```python
from build123d import *

# Parameters (mm, degrees)
ESQUISSE1_W        = 20
ESQUISSE1_H        = 5
BOSS_EXTRU_1_DEPTH = 5


with BuildPart() as part:
    # Esquisse1 → Boss.-Extru.1 (new body)
    with BuildSketch(Plane.XY):
        Polygon((-100, 150), (100, 150), (100, 75), (105, 75), (105, 150), (113, 150), (113, 0), (-113, 0), (-113, 150), (-105, 150), (-105, 75), (-100, 75), align=None)
        with Locations((83, 7.5)):
            Rectangle(ESQUISSE1_W, ESQUISSE1_H, mode=Mode.SUBTRACT)
        with Locations((83, 57.5)):
            Rectangle(ESQUISSE1_W, ESQUISSE1_H, mode=Mode.SUBTRACT)
        Polygon((-15, 5), (15, 5), (15, 10), (0, 10), (-15, 10), align=None, mode=Mode.SUBTRACT)
        Polygon((-15, 60), (0, 60), (15, 60), (15, 55), (-15, 55), align=None, mode=Mode.SUBTRACT)
        with Locations((-83, 7.5)):
            Rectangle(ESQUISSE1_W, ESQUISSE1_H, mode=Mode.SUBTRACT)
        with Locations((-83, 57.5)):
            Rectangle(ESQUISSE1_W, ESQUISSE1_H, mode=Mode.SUBTRACT)
    extrude(amount=BOSS_EXTRU_1_DEPTH)


solid = part.part
```
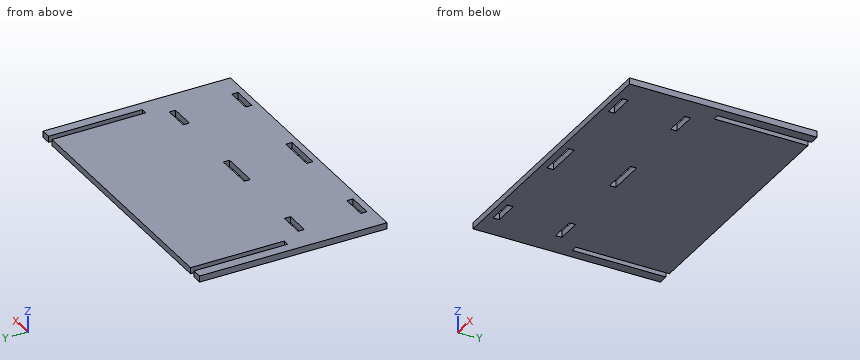
The model under review builds one solid part; all positions refer to its coordinate system, in mm. Round coordinates to 2 decimals unless told otherwise and drop trailing zeros. Loops run counter-clockwise (first coordinate to the right, second up) from the corner with the lowest first, then second, coordinate; pieces in that order, holes last. Notation, with made-up numbers: M 55.5,56.5 L 60.5,56.5 A30 ccw 60.5,90.5 Z; hole C 68.25,-16.75 d3. An arc over 180 degrees is marked long. Answer as a JSON object with one key per item and string values.
(1) Take a section at B-B on x = 83.5. Give the boundary of the cut face in (y, z), and give its area (3 significant figures).
Resolved:
{"outline": "M 0,0 L 5,0 L 5,5 L 0,5 Z; M 10,0 L 55,0 L 55,5 L 10,5 Z; M 60,0 L 150,0 L 150,5 L 60,5 Z", "area": "700 mm²"}
(2) Take a section at A-A on y = 114. Give the boundary of the cut face in (x, z).
Resolved:
{"outline": "M -113,0 L -105,0 L -105,5 L -113,5 Z; M -100,0 L 100,0 L 100,5 L -100,5 Z; M 105,0 L 113,0 L 113,5 L 105,5 Z"}
(3) To check wall thickness, follow line 1 along X through (y, z) = (59, 1.5); line 2 along Y through (x, z) = (9, 1.2); line 3 along X through (y, z) = (115, 0.6). State the ranges of each line that lie inside material, in increasing order.
Resolved:
{"line 1": "-113 to -93, -73 to -15, 15 to 73, 93 to 113", "line 2": "0 to 5, 10 to 55, 60 to 150", "line 3": "-113 to -105, -100 to 100, 105 to 113"}
(4) Take a section at C-C on z = 2.2. Count the separate pieces of the cut face and the enclosed holes in it, and give its area (4 significant figures).
Resolved:
{"separate pieces": "1", "enclosed holes": "6", "area": "32,450 mm²"}
